```python
from build123d import *

# Parameters (mm, degrees)
SKETCH1_W           = 41.5
SKETCH1_H           = 21
SKETCH1_W_2         = 21
SKETCH1_H_2         = 41.5
BOSS_EXTRUDE1_DEPTH = 5


with BuildPart() as part:
    # Sketch1 → Boss-Extrude1 (new body)
    with BuildSketch(Plane.XY):
        Polygon((105, 43.492424049), (43.492424049, 105), (-43.492424049, 105), (-105, 43.492424049), (-105, -43.492424049), (-43.492424049, -105), (43.492424049, -105), (105, -43.492424049), align=None)
        Polygon((47.022600949, -32.173358544), (76.367532368, -61.518289963), (61.518289963, -76.367532368), (32.173358544, -47.022600949), align=None, mode=Mode.SUBTRACT)
        with Locations((76.75, 0)):
            Rectangle(SKETCH1_W, SKETCH1_H, mode=Mode.SUBTRACT)
        with Locations((0, -76.75)):
            Rectangle(SKETCH1_W_2, SKETCH1_H_2, mode=Mode.SUBTRACT)
        Polygon((-32.173358544, -47.022600949), (-61.518289963, -76.367532368), (-76.367532368, -61.518289963), (-47.022600949, -32.173358544), align=None, mode=Mode.SUBTRACT)
        with Locations((-76.75, 0)):
            Rectangle(SKETCH1_W, SKETCH1_H, mode=Mode.SUBTRACT)
        Polygon((-47.022600949, 32.173358544), (-76.367532368, 61.518289963), (-61.518289963, 76.367532368), (-32.173358544, 47.022600949), align=None, mode=Mode.SUBTRACT)
        with Locations((0, 76.75)):
            Rectangle(SKETCH1_W_2, SKETCH1_H_2, mode=Mode.SUBTRACT)
        Polygon((32.173358544, 47.022600949), (61.518289963, 76.367532368), (76.367532368, 61.518289963), (47.022600949, 32.173358544), align=None, mode=Mode.SUBTRACT)
    extrude(amount=BOSS_EXTRUDE1_DEPTH)


solid = part.part
```
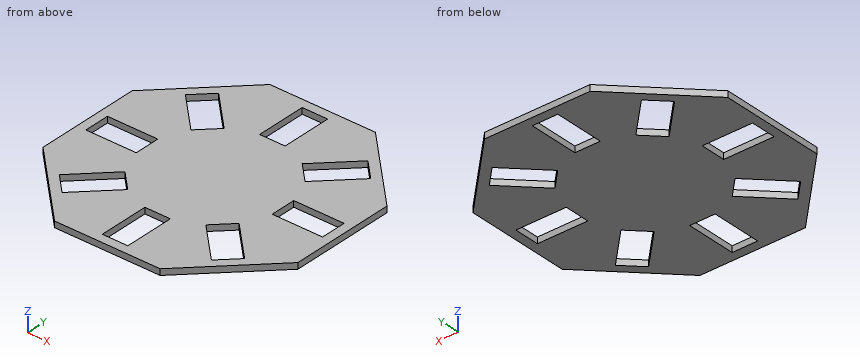
Model file for the job. Use its own axes, mm. Coordinates: 2 decimals unless noted, no trailing zeros. Loops run counter-clockwise (first coordinate to the right, second up) from the corner with the lowest first, then second, coordinate; pieces in that order, holes last. Notation, with made-up numbers: M 35.25,3.25 L 49.25,3.25 A15 ccw 49.25,28.25 Z; hole C -29,64 d2. An arc over 180 degrees is marked long. Use CSV: the item, a comma, the result in double quotes. Start each with the question number.
1. Band-saw the part on D-D, the plane z = 3. Give the number of separate pieces and of enclosed holes in the cut face, then the cut area to 3 significant figures.
2. Band-saw the part on A-A, the plane x = -65. List the corners of the cut face in (y, z), then the cut area to 3 significant figures.
3. Band-saw the part on C-C, the plane x = 85.5. List the corners of the cut face in (y, z), then the cut area to 3 significant figures.
4. Flat gauge pins, fed straight in: pin 1 (2.5 mm diameter, centred on x = 79, z = 3, fed in from -Y); pin 2 (1.5 mm diameter, centred on y = 74, z = 2.5, fed in from +X); pin 3 (2.5 mm diameter, centred on y = -77.5, z = 1.5, fed in from +X). Where does each tip first touch, or does it go through?
5. Band-saw the part on B-B, the plane y = -38. List the corners of the cut face in (x, z), then the cut area to 3 significant figures.
6. Probe probe 1 along Y at (x, z) = (0.5, 1.45); probe 2 along X at (y, z) = (62, 2.75). List the from-to ranges inside material, lowest first. Write a range as [from, to].
Entries:
1,separate pieces,"1"
1,enclosed holes,"8"
1,area,"29,600 mm2"
2,outline,"M -83.49,0 L -72.89,0 L -72.89,5 L -83.49,5 Z; M -50.15,0 L -10.5,0 L -10.5,5 L -50.15,5 Z; M 10.5,0 L 50.15,0 L 50.15,5 L 10.5,5 Z; M 72.89,0 L 83.49,0 L 83.49,5 L 72.89,5 Z"
2,area,"503 mm2"
3,outline,"M -62.99,0 L -10.5,0 L -10.5,5 L -62.99,5 Z; M 10.5,0 L 62.99,0 L 62.99,5 L 10.5,5 Z"
3,area,"525 mm2"
4,pin 1,"stops at y = -70.74"
4,pin 2,"stops at x = 75.24"
4,pin 3,"stops at x = 72.24"
5,outline,"M -105,0 L -52.85,0 L -52.85,5 L -105,5 Z; M -41.2,0 L 41.2,0 L 41.2,5 L -41.2,5 Z; M 52.85,0 L 105,0 L 105,5 L 52.85,5 Z"
5,area,"933 mm2"
6,probe 1,"y = [-105, -97.5], [-56, 56], [97.5, 105]"
6,probe 2,"x = [-86.49, -75.89], [-47.15, -10.5], [10.5, 47.15], [75.89, 86.49]"
